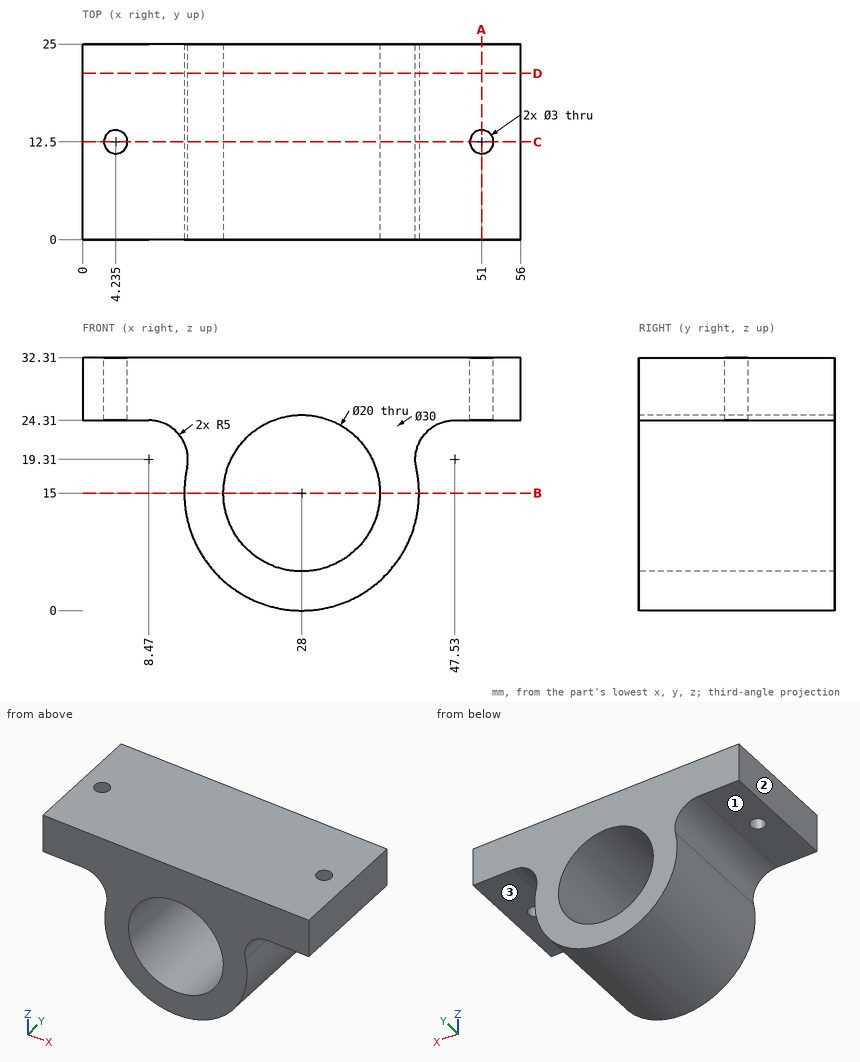
The figure shows three views and two pictorial views of one solid part (mm, origin at its lowest corner). Answer the questions. A direction names the side the tool comes from. Round coordinates to 2 decimals unless told otherwise and drop trailing zeros. Loops run counter-clockwise (first coordinate to the right, second up) from the corner with the lowest first, then second, coordinate; pieces in that order, holes last. Notation, with made-up numbers: (47, -6.5) - (84, -6.5) arc R22 cw to (84, 3.5) - close; hole circle Ø7 at (34, 89). An arc over 180 degrees is marked (long way). One line per question, with ' | ' between items. Start each with the question number.
Q1. Section C-C on y = 12.5 is taken. Give the vertices of the cut face in (x, z) (1 decimal), plus the area to 3 significant figures.
Q2. Flat-ended cylindrical pins translate along their axes: pin 1 (1.5 mm diameter, centred on x = 39, y = 20.5, fed in from -Z); pin 2 (2.5 mm diameter, centred on x = 2.5, y = 18, fed in from -Z); pin 3 (10 mm diameter, centred on y = 17, z = 11, fed in from +X). Find the tip coordinate at first contact, or state that the pin passes through.
Q3. For the marked faces 1, 2 and 3, determine the directions among +Z, -Z, +X, -X, +Y, -Y from which every point of the face is accessible in a straight line to the end or side of a thin tool.
Q4. Section B-B on z = 15 is taken. Give the vertices of the cut face in (x, y).
Q5. Section A-A on x = 51 is taken. Give the vertices of the cut face in (y, z).
Q6. Find the intervals of material crossed by L1, parallel to X at y = 15.25, z = 15; L2, parallel to Y at x = 51, z = 28; L3, parallel to X at y = 13, z = 28.5, in increasing order.
Q7. Section D-D on y = 21.25 is taken. Give the vertices of the cut face in (x, z).
Established:
1) outline: (0, 24.3) - (2.7, 24.3) - (2.7, 32.3) - (0, 32.3) - close; (5.7, 24.3) - (8.5, 24.3) arc R5 cw to (13.4, 18.2) arc R15 ccw (long way) to (42.6, 18.2) arc R5 cw to (47.5, 24.3) - (49.5, 24.3) - (49.5, 32.3) - (5.7, 32.3) - close; (52.5, 24.3) - (56, 24.3) - (56, 32.3) - (52.5, 32.3) - close; hole circle Ø20 at (28, 15) | area: 723 mm²
2) pin 1: z = 4.05 | pin 2: z = 24.31 | pin 3: x = 43
3) face 1: -Z, -X, +Y, -Y | face 2: +Z, -Z, -X, +Y, -Y | face 3: -Z, +X, +Y, -Y
4) outline: (13, 0) - (18, 0) - (18, 25) - (13, 25) - close; (38, 0) - (43, 0) - (43, 25) - (38, 25) - close
5) outline: (0, 24.31) - (11, 24.31) - (11, 32.31) - (0, 32.31) - close; (14, 24.31) - (25, 24.31) - (25, 32.31) - (14, 32.31) - close
6) L1: 13 to 18, 38 to 43 | L2: 0 to 11, 14 to 25 | L3: 0 to 2.82, 5.65 to 49.59, 52.41 to 56
7) outline: (0, 24.31) - (8.47, 24.31) arc R5 cw to (13.35, 18.23) arc R15 ccw (long way) to (42.65, 18.23) arc R5 cw to (47.53, 24.31) - (56, 24.31) - (56, 32.31) - (0, 32.31) - close; hole circle Ø20 at (28, 15)
